Can you work these out from the model? Positions are in its coordinate system, mm. A direction names the side the tool comes from. Give positions to 0.01 mm unless a question says otherwise; leave off trailing zeros. Loops run counter-clockwise (first coordinate to the right, second up) from the corner with the lowest first, then second, coordinate; pieces in that order, holes last. Notation, with made-up numbers: M -20.75,7.5 L 11.25,7.5 A23 cw 11.25,32.5 Z; hole C -13.5,50 d6. An arc over 180 degrees is marked long. Put each result on its own line as item: value. Start each with the question number.
1) For faces 4 (the cylindrical face through (-9.46, -47.56, 32.53)), 5 (the flat face through (0, -20, -30)), 6 (the flat face through (-3.92, -22.03, -37.53)), 7 (the flat face through (-4, -55, 32)), 8 (the flat face through (-12.03, -31.42, 37.53)), which set-ups out of +Z, -Z, +X, -X, +Y, -Y let a thin tool reach every point of the face, with its end or its side?
2) Please list where these lines run through material, in increasing order: line 1 along Z through (x, y) = (-15, -22); line 2 along X through (y, z) = (-20, 32.5); line 3 along X through (y, z) = (-35, 31.95). Write a range as from..to.
3) Imagine slicing it at C-C (y = -35). Write out the boundary of the cut face in (x, z).
4) If we mould it in two halves opening along Y, with no side actions, what happens to faces 1 (the flat face through (20, -7, -1)), 2 (the flat face through (0, -10, -2)), 3 (the flat face through (-5, -22, -35))? For each: +Y half, -Y half, draft (parallel to the pull), parting line (faces both ways), or undercut.
5) Imagine slicing it at D-D (x = 7.5). State how many separate pieces and enclosed holes the cut face has, then the cut area to 3 significant figures.
6) Imagine slicing it at B-B (z = 0). Write out the boundary of the cut face in (x, y), then the cut area to 3 significant figures.
7) Imagine slicing it at A-A (x = 0). Write out the boundary of the cut face in (y, z), then the cut area to 3 significant figures.
8) For P1, Ø5.5, axis at y = -56.5, z = 32.5, coming from the +X side; P2, Ø4.5, axis at x = 29.5, z = 35, coming from the +Y side; P3, Ø1.4, axis at y = -49.5, z = 37, coming from the +X side; P4, Ø2, axis at x = 13, z = -21.5, coming from the -Y side, each with a flat end and sliding along its axis, tell me the tip position at first contact or that it passes through.
from build123d import *

# Parameters (mm, degrees)
SKETCH_W        = 40
SKETCH_H        = 80
PAD_DEPTH       = 10
SKETCH001_W     = 40
SKETCH001_H     = 10
PAD001_DEPTH    = 50
SKETCH002_R     = 2.5
POCKET_DEPTH    = 10
SKETCH003_R     = 2.5
POCKET001_DEPTH = 10
POCKET002_DEPTH = 5
SKETCH006_R     = 2.5
POCKET003_DEPTH = 84
SKETCH008_W     = 40
SKETCH008_H     = 30
POCKET005_DEPTH = 10
SKETCH010_W     = 10
SKETCH010_H     = 30
PAD002_DEPTH    = 13
POCKET006_DEPTH = 12
POCKET007_DEPTH = 5
SKETCH013_W     = 5
SKETCH013_H     = 10
POCKET008_DEPTH = 37
CHAMFER_SIZE    = 4


with BuildPart() as part:
    # Sketch → Pad (new body)
    with BuildSketch(Plane.XZ):
        Rectangle(SKETCH_W, SKETCH_H)
    extrude(amount=PAD_DEPTH)

    # Sketch001 (on Face6 of Pad) → Pad001 (join)
    with BuildSketch(Plane.XZ.offset(10)):
        with Locations((0, 35)):
            Rectangle(SKETCH001_W, SKETCH001_H)
        with Locations((0, -35)):
            Rectangle(SKETCH001_W, SKETCH001_H)
    extrude(amount=PAD001_DEPTH)

    # Sketch002 (on Face8 of Pad001) → Pocket (cut)
    with BuildSketch(Plane.XZ.offset(10)):
        with Locations((-7.5, 0)):
            Circle(SKETCH002_R)
        with Locations((7.5, 0)):
            Circle(SKETCH002_R)
    extrude(amount=-POCKET_DEPTH, mode=Mode.SUBTRACT)

    # Sketch003 (on Face5 of Pocket) → Pocket001 (cut)
    with BuildSketch(Plane(origin=(0, 0, 40), x_dir=(-1, 0, 0), z_dir=(0, 0, 1))):
        with Locations((10, 50)):
            Circle(SKETCH003_R)
        with Locations((10, 35)):
            Circle(SKETCH003_R)
    extrude(amount=-POCKET001_DEPTH, mode=Mode.SUBTRACT)

    # Sketch004 (on Face5 of Pocket001) → Pocket002 (cut)
    with BuildSketch(Plane(origin=(0, 0, 40), x_dir=(-1, 0, 0), z_dir=(0, 0, 1))):
        Polygon((14.113621, 47.625), (14.113621, 52.375), (10, 54.75), (5.886379, 52.375), (5.886379, 47.625), (10, 45.25), align=None)
        Polygon((14.113621, 32.625), (14.113621, 37.375), (10, 39.75), (5.886379, 37.375), (5.886379, 32.625), (10, 30.25), align=None)
    extrude(amount=-POCKET002_DEPTH, mode=Mode.SUBTRACT)

    # Sketch006 (on Face27 of Pocket002) → Pocket003 (cut)
    with BuildSketch(Plane(origin=(0, 0, -40), x_dir=(1, 0, 0), z_dir=(0, 0, -1))):
        with Locations((-7.5, 20)):
            Circle(SKETCH006_R)
        with Locations((7.5, 20)):
            Circle(SKETCH006_R)
    extrude(amount=-POCKET003_DEPTH, mode=Mode.SUBTRACT)

    # Sketch008 → Pocket005 (cut)
    with BuildSketch(Plane(origin=(0, 0, -40), x_dir=(1, 0, 0), z_dir=(0, 0, -1))):
        with Locations((0, 45)):
            Rectangle(SKETCH008_W, SKETCH008_H)
    extrude(amount=-POCKET005_DEPTH, mode=Mode.SUBTRACT)

    # Sketch010 → Pad002 (join)
    with BuildSketch(Plane(origin=(20, 0, 0), x_dir=(0, 0, 1), z_dir=(1, 0, 0))):
        with Locations((35, 45)):
            Rectangle(SKETCH010_W, SKETCH010_H)
    extrude(amount=PAD002_DEPTH)

    # Sketch011 → Pocket006 (cut)
    with BuildSketch(Plane(origin=(0, 0, 0), x_dir=(1, 0, 0), z_dir=(0, 1, 0))):
        with BuildLine():
            ThreePointArc((-9, 30), (0, 21), (9, 30))
            Line((9, 30), (9, 50))
            ThreePointArc((9, 50), (0, 59), (-9, 50))
            Line((-9, 50), (-9, 30))
        make_face()
    extrude(amount=-POCKET006_DEPTH, mode=Mode.SUBTRACT)

    # Sketch012 (on Face34 of Pocket006) → Pocket007 (cut)
    with BuildSketch(Plane(origin=(0, 0, -40), x_dir=(1, 0, 0), z_dir=(0, 0, -1))):
        Polygon((-2.75, 20), (-5.125, 24.113621), (-9.875, 24.113621), (-12.25, 20), (-9.875, 15.886379), (-5.125, 15.886379), align=None)
        Polygon((9.875, 15.886379), (12.25, 20), (9.875, 24.113621), (5.125, 24.113621), (2.75, 20), (5.125, 15.886379), align=None)
    extrude(amount=-POCKET007_DEPTH, mode=Mode.SUBTRACT)

    # Sketch013 (on Face41 of Pocket007) → Pocket008 (cut)
    with BuildSketch(Plane(origin=(33, 0, 0), x_dir=(0, 0, 1), z_dir=(1, 0, 0))):
        with Locations((32.5, 55)):
            Rectangle(SKETCH013_W, SKETCH013_H)
    extrude(amount=-POCKET008_DEPTH, mode=Mode.SUBTRACT)

    # Chamfer
    chamfer_edges = [part.edges().sort_by_distance(p)[0] for p in [
        (0, -10, 30),
        (20, -30, 35),
        (0, -60, 40),
        (26.5, -60, 40),
        (33, -45, 40),
        (20, -30, -35),
        (-20, -30, -35),
    ]]
    chamfer(chamfer_edges, length=CHAMFER_SIZE)


solid = part.part
Recorded:
1. face 4: +Z, -Z
1. face 5: +X, -X, -Y
1. face 6: -Z
1. face 7: -Z, +X, -Y
1. face 8: +Z
2. line 1: -40..-30, 30..40
2. line 2: -20..-10, -5..5, 10..20
2. line 3: -20..-12.5, -7.5..33
3. outline: M -20,30 L -12.5,30 L -12.5,35 L -14.11,35 L -14.11,40 L -20,40 Z; M -7.5,30 L 33,30 L 33,36 L 29,40 L -5.89,40 L -5.89,35 L -7.5,35 Z
4. face 1: draft
4. face 2: -Y half
4. face 3: undercut
5. separate pieces: 5
5. enclosed holes: 0
5. area: 1,110 mm²
6. outline: M -20,-10 L -10,-10 L -10,0 L -20,0 Z; M -5,-10 L 5,-10 L 5,0 L -5,0 Z; M 10,-10 L 20,-10 L 20,0 L 10,0 Z
6. area: 300 mm²
7. outline: M -60,35 L -50,35 L -50,30 L -14,30 L -10,26 L -10,-21 L 0,-21 L 0,40 L -56,40 L -60,36 Z; M -30,-40 L -12,-40 L -12,-30 L -30,-30 Z
7. area: 1,240 mm²
8. P1: x = 33
8. P2: y = -30
8. P3: x = 32.7
8. P4: y = -10
